```python
from build123d import *

# Parameters (mm, degrees)
SKETCH2_R           = 2.95
SKETCH2_R_2         = 1.55
BOSS_EXTRUDE1_DEPTH = 34.8
CHAMFER3_SIZE       = 0.4
CHAMFER4_SIZE       = 0.4


with BuildPart() as part:
    # Sketch2 → Boss-Extrude1 (new body)
    with BuildSketch(Plane(origin=(0, 0, 0), x_dir=(1, 0, 0), z_dir=(0, 1, 0))):
        with Locations(Location((0, 0, 0), (0, 0, 270))):
            Circle(SKETCH2_R)
        with Locations(Location((0, 0, 0), (0, 0, 270))):
            Circle(SKETCH2_R_2, mode=Mode.SUBTRACT)
    extrude(amount=BOSS_EXTRUDE1_DEPTH)

    # Chamfer3
    chamfer3_edges = [part.edges().sort_by_distance(p)[0] for p in [
        (0, 0, -2.95),
    ]]
    chamfer(chamfer3_edges, length=CHAMFER3_SIZE)

    # Chamfer4
    chamfer4_edges = [part.edges().sort_by_distance(p)[0] for p in [
        (0, 34.8, -2.95),
    ]]
    chamfer(chamfer4_edges, length=CHAMFER4_SIZE)


solid = part.part
```
Here's how the part is built. I have some questions about the finished solid (model axes, mm). Give positions to 0.01 mm unless a question says otherwise; leave off trailing zeros. Loops run counter-clockwise (first coordinate to the right, second up) from the corner with the lowest first, then second, coordinate; pieces in that order, holes last. Notation, with made-up numbers: M 11.5,-17 L 51.5,-17 A12 ccw 51.5,-2 Z; hole C 20,-15 d3. An arc over 180 degrees is marked long. Return JSON: item names as keys, results as strings.
Item 1: Thinking about a two-plate mould opening in X: for faces 1 (the cylindrical face through (-2.88, 17.16, -0.64)), 2 (the flat face through (0, 34.8, 2)), 3 (the cylindrical face through (0.466, 17.156, 1.478)), which applies, released by +X, released by -X, zero draft, split by the parting line, or undercut?
A:
{"face 1": "split by the parting line", "face 2": "zero draft", "face 3": "undercut"}
Item 2: Imagine slicing it at B-B on z = 0. List the corners of the cut face in (x, y) for me, then the cut area to 3 significant figures.
A:
{"outline": "M -2.95,0.4 L -2.55,0 L -1.55,0 L -1.55,34.8 L -2.55,34.8 L -2.95,34.4 Z; M 1.55,0 L 2.55,0 L 2.95,0.4 L 2.95,34.4 L 2.55,34.8 L 1.55,34.8 Z", "area": "97.1 mm^2"}
Item 3: Please list where these lines run through material, in increasing order: line 1 (X direction, y = 13, z = 0); line 2 (X direction, y = 21, z = 1.2).
A:
{"line 1": "x = -2.95 to -1.55, 1.55 to 2.95", "line 2": "x = -2.69 to -0.98, 0.98 to 2.69"}
Item 4: Imagine slicing it at C-C on y = 24. List the corners of the cut face in (x, z) for me, then the cut area to 3 significant figures.
A:
{"outline": "C 0,0 d5.9; hole C 0,0 d3.1", "area": "19.8 mm^2"}
Item 5: Imagine slicing it at A-A on x = 0. List the corners of the cut face in (y, z) for me, then the cut area to 3 significant figures.
A:
{"outline": "M 0,-2.55 L 0.4,-2.95 L 34.4,-2.95 L 34.8,-2.55 L 34.8,-1.55 L 0,-1.55 Z; M 0,1.55 L 34.8,1.55 L 34.8,2.55 L 34.4,2.95 L 0.4,2.95 L 0,2.55 Z", "area": "97.1 mm^2"}
Item 6: I'm going to push flat-ended pins straight in: pin 1 Ø3 at (x, y) = (-1, 5) entering from +Z; pin 2 Ø2 at (x, y) = (-2.5, 14) entering from -Z. Where does each tip first touch, or does it pass through?
A:
{"pin 1": "stops at z = 2.95", "pin 2": "stops at z = -2.54"}
